from build123d import *

# Parameters (mm, degrees)
SKICA1_W                 = 40
SKICA1_H                 = 10
P_IDAT_VYSUNUT_M1_DEPTH  = 5
SKICA2_R                 = 1.65
ODEBRAT_VYSUNUT_M1_DEPTH = 5
ZAOBLIT2_R               = 5
SKICA3_R                 = 1.65
ODEBRAT_VYSUNUT_M2_DEPTH = 10


with BuildPart() as part:
    # Skica1 → Přidat vysunutím1 (new body)
    with BuildSketch(Plane.XY):
        with Locations((20, 5)):
            Rectangle(SKICA1_W, SKICA1_H)
    extrude(amount=P_IDAT_VYSUNUT_M1_DEPTH)

    # Skica2 → Odebrat vysunutím1 (cut)
    with BuildSketch(Plane.XY.offset(5)):
        with Locations((5, 5)):
            Circle(SKICA2_R)
        with Locations((35, 5)):
            Circle(SKICA2_R)
    extrude(amount=-ODEBRAT_VYSUNUT_M1_DEPTH, mode=Mode.SUBTRACT)

    # Zaoblit2
    zaoblit2_edges = [part.edges().sort_by_distance(p)[0] for p in [
        (40, 0, 2.5),
        (40, 10, 2.5),
        (0, 0, 2.5),
        (0, 10, 2.5),
    ]]
    fillet(zaoblit2_edges, radius=ZAOBLIT2_R - 0.0001)  # a hair under: the kernel refuses the full size

    # Skica3 → Odebrat vysunutím2 (cut)
    with BuildSketch(Plane.XY.offset(5)):
        with Locations((25, 5)):
            Circle(SKICA3_R)
    extrude(amount=-ODEBRAT_VYSUNUT_M2_DEPTH, mode=Mode.SUBTRACT)


solid = part.part
Geometry check sheet. Reference: the model listing, model coordinates, mm. Give positions to 0.01 mm unless a question says otherwise; leave off trailing zeros. Write each loop counter-clockwise with the first axis right and the second up, starting at its lowest first coordinate (ties: lowest second). Pieces come first, ordered by that corner, then holes. Notation, with made-up numbers: M -12,44 L 11,44 A32 cw 11,78 Z; hole C 67.5,39 d2. An arc over 180 degrees is marked long. Answer as CSV lines item,"result". Start each with the question number.
Q1. Release check for a two-part mould opening along Y. For faces 1 (the face through (20, 5, 0)), 2 (the face through (23.35, 5.07, 2.54)), 3 (the face through (38, 1, 3)) record: pulls with the +Y half, pulls with the -Y half, needs draft (parallel to the pull), parting line crosses it, or undercut.
Q2. Material ranges on L1, parallel to Y at x = 35, z = 2.35; L2, parallel to X at y = 5.75, z = 1.1; L3, parallel to X at y = 6.5, z = 2.2, recorded low to high.
Q3. Section check B-B, the plane z = 2.95. Give the number of separate pieces and of enclosed holes in the cut face, then the cut area to 3 significant figures.
Q4. Section check C-C, the plane y = 5.75. Record the cut outline in (x, z).
Q5. Section check D-D, the plane x = 4. Record the cut outline in (y, z), then the cut area to 3 significant figures.
Q6. Go/stop test with a flat-tipped pin: pin 1 (2 mm diameter, centred on x = 5, y = 5, fed in from +Z). Record where the tip stops, or that it passes through.
Q7. Section check A-A, the plane x = 25. Record the cut outline in (y, z).
Geometry says:
1,face 1,"needs draft"
1,face 2,"undercut"
1,face 3,"pulls with the -Y half"
2,L1,"0 to 3.35, 6.65 to 10"
2,L2,"0.06 to 3.53, 6.47 to 23.53, 26.47 to 33.53, 36.47 to 39.94"
2,L3,"0.23 to 4.31, 5.69 to 24.31, 25.69 to 34.31, 35.69 to 39.77"
3,separate pieces,"1"
3,enclosed holes,"3"
3,area,"353 mm^2"
4,outline,"M 0.06,0 L 3.53,0 L 3.53,5 L 0.06,5 Z; M 6.47,0 L 23.53,0 L 23.53,5 L 6.47,5 Z; M 26.47,0 L 33.53,0 L 33.53,5 L 26.47,5 Z; M 36.47,0 L 39.94,0 L 39.94,5 L 36.47,5 Z"
5,outline,"M 0.1,0 L 3.69,0 L 3.69,5 L 0.1,5 Z; M 6.31,0 L 9.9,0 L 9.9,5 L 6.31,5 Z"
5,area,"35.9 mm^2"
6,pin 1,"through"
7,outline,"M 0,0 L 3.35,0 L 3.35,5 L 0,5 Z; M 6.65,0 L 10,0 L 10,5 L 6.65,5 Z"
